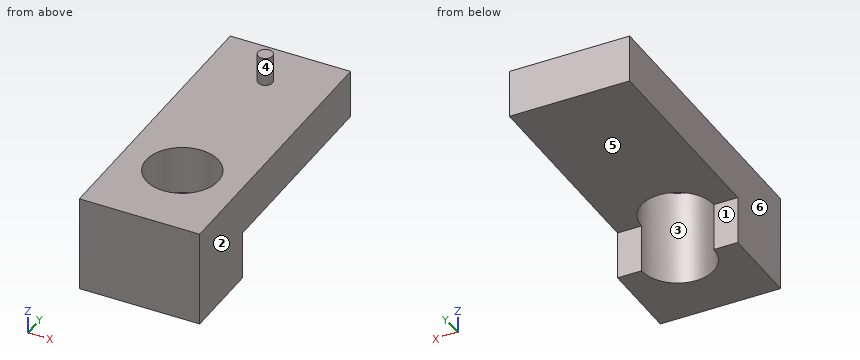
Autodesk Inventor part; units mm, degrees
ref_plane "YZ Plane" through (0, 0, 0) normal (1, 0, 0) x (0, 1, 0)
ref_plane "XZ Plane" through (0, 0, 0) normal (0, 1, 0) x (-1, 0, 0)
ref_plane "XY Plane" through (0, 0, 0) normal (0, 0, 1) x (1, 0, 0)
sketch "Sketch1" plane through (0, 0, 0) normal (0, 0, 1) x (1, 0, 0)
  line L0 (-12.5, -12.5) -> (12.5, -12.5)
  line L1 (12.5, -12.5) -> (12.5, 47.5)
  line L2 (12.5, 47.5) -> (-12.5, 47.5)
  line L3 (-12.5, 47.5) -> (-12.5, -12.5)
  point P0 (0, 0)
  dimension "d0" = 60
  dimension "d1" = 25
  dimension "d2" = 12.5
  dimension "d5" = 12.5
extrude "Extrusion1" add sketch "Sketch1" against normal blind 10
sketch "Sketch2" plane through (0, 0, 0) normal (0, 0, 1) x (1, 0, 0)
  circle A0 centre (0, 37.5) radius 1.5
  point P0 (0, 0)
  dimension "d8" = 3
  dimension "d29" = 37.5
extrude "Extrusion2" add sketch "Sketch2" along normal blind 6
thread "Thread1"
sketch "Sketch3" plane through (0, 0, -10) normal (0, 0, -1) x (-1, 0, 0)
  line L0 (-7.5, 4.5) -> (-12.5, 4.5)
  line L1 (-12.5, 47.5) -> (-12.5, -12.5)
  line L2 (-12.5, -12.5) -> (12.5, -12.5)
  line L3 (-12.5, -12.5) -> (12.5, -12.5)
  line L4 (12.5, -12.5) -> (12.5, 4.5)
  line L5 (12.5, -12.5) -> (12.5, 47.5)
  line L6 (7.5, 4.5) -> (12.5, 4.5)
  arc A0 (-7.5, 4.5) -> (7.5, 4.5) centre (0, 4.5) ccw
  point P0 (0, 0)
  dimension "d20" = 17
  dimension "d21" = 5
  dimension "d22" = 5
  dimension "d25" = 7.5
extrude "Extrusion3" add sketch "Sketch3" along normal blind 10
sketch "Sketch5" plane through (0, 0, 0) normal (0, 0, 1) x (1, 0, 0)
  circle A0 centre (0, 4.5) radius 7.5
  point P0 (0, 0)
  dimension "d26" = 15
extrude "Extrusion5" cut sketch "Sketch5" against normal blind 10
properties part number "bottom_part"
Model file for the job. Use its own axes, mm. Face numbers are marked on the shaded views. A direction names the side the tool comes from. Give positions to 0.01 mm unless a question says otherwise; leave off trailing zeros. Loops run counter-clockwise (first coordinate to the right, second up) from the corner with the lowest first, then second, coordinate; pieces in that order, holes last. Notation, with made-up numbers: (23.25, 48) - (74.25, 48) arc R28 ccw to (74.25, 80) - close; hole circle Ø3 at (44, 36.25). An arc over 180 degrees is marked (long way). One line per item, written item: value. Start each with the question number.
1. Slice it at B-B (y = 37.5). List the corners of the cut face in (x, z).
2. Pull direction X, two halves, no side cores. Call the marked faces 3, 4, 5 and 6: pulls with the +X half, pulls with the -X half, needs draft (parallel to the pull), parting line crosses it, or undercut.
3. Which spindle directions (+Z, -Z, +X, -X, +Y, -Y) get a long thin tool onto all of the face, cutting with end or side? Do the marked faces 1 and 2. Say none if no direction does.
4. Probe L1, parallel to X at y = 4.5, z = -5; L2, parallel to Y at x = 0, z = -8.5; L3, parallel to Z at x = 1, y = 32. List the from-to ranges inside material, lowest first. Write a range as from..to.
5. Slice it at D-D (y = 3). List the corners of the cut face in (x, z), plus the area to 3 significant figures.
6. Slice it at A-A (z = -9.25). List the corners of the cut face in (x, y), plus the area to 3 significant figures.
7. Pin check, flat tips, straight feed: pin 1 (1.5 mm diameter, centred on x = 7.5, y = 31, fed in from +Z); pin 2 (1.5 mm diameter, centred on x = -9.5, z = -12.5, fed in from +Y); pin 3 (6 mm diameter, centred on x = 8.5, y = 36, fed in from -Z). Stop position of each tip, or through.
8. Slice it at C-C (x = 0.5). List the corners of the cut face in (y, z), plus the area to 3 significant figures.
Solution:
1. outline: (-12.5, -10) - (12.5, -10) - (12.5, 0) - (1.5, 0) - (1.5, 6) - (-1.5, 6) - (-1.5, 0) - (-12.5, 0) - close
2. face 3: undercut
2. face 4: parting line crosses it
2. face 5: needs draft
2. face 6: pulls with the -X half
3. face 1: -Z, +X, -X, +Y
3. face 2: +Z, -Z, +X, +Y, -Y
4. L1: x = -12.5..-7.5, 7.5..12.5
4. L2: y = -12.5..-3, 12..47.5
4. L3: z = -10..0
5. outline: (-12.5, -20) - (-7.35, -20) - (-7.35, 0) - (-12.5, 0) - close; (7.35, -20) - (12.5, -20) - (12.5, 0) - (7.35, 0) - close
5. area: 206 mm^2
6. outline: (-12.5, -12.5) - (12.5, -12.5) - (12.5, 47.5) - (-12.5, 47.5) - close; hole circle Ø15 at (0, 4.5)
6. area: 1,320 mm^2
7. pin 1: stops at z = 0
7. pin 2: stops at y = 4.5
7. pin 3: stops at z = -10
8. outline: (-12.5, -20) - (-2.98, -20) - (-2.98, 0) - (-12.5, 0) - close; (11.98, -10) - (47.5, -10) - (47.5, 0) - (38.91, 0) - (38.91, 6) - (36.09, 6) - (36.09, 0) - (11.98, 0) - close
8. area: 562 mm^2
